Read the model definition and answer for the solid it produces. Units are mm, in the model's axes. A direction names the side the tool comes from. Coordinates: 2 decimals unless noted, no trailing zeros. Write each loop counter-clockwise with the first axis right and the second up, starting at its lowest first coordinate (ties: lowest second). Pieces come first, ordered by that corner, then holes.
(1) Find the intervals of material crossed by probe 1 along X at (y, z) = (-1.5, -0.05); probe 2 along X at (y, z) = (1, -0.35); probe 3 along Z at (x, y) = (-9, -0.5), in increasing order.
(2) Section B-B on y = 1 is taken. Write down the section's boundary in (x, z).
(3) Which of the six approach directions +Z, -Z, +X, -X, +Y, -Y give full straight-line access (tool end or side, diameter ignored) to faces 1 (the flat face through (0, 0, 0)), 2 (the flat face through (0, 0, 1.2))?
(4) Given pin 1 (1.5 mm diameter, centred on x = -18.08, y = 0.47, fed in from +Z), flat-ended and moving along its own axis, determine where the tip first touches the part or whether it passes through.
(5) Section A-A on y = -1.25 is taken. Write down the section's boundary in (x, z), then the cut area to 3 significant figures.
(6) The mould has two halves that part along X. Classify faces 3 (the cylindrical face through (0.295, -4.139, 0.858)), 4 (the cylindrical face through (19.324, 0.525, 0.338)), 5 (the flat face through (-21.5, 0, 0)), 6 (the flat face through (21.5, 0, 0)): +X half, -X half, draft (parallel to the pull), parting line (faces both ways), or undercut.
from build123d import *

# Parameters (mm, degrees)
ESBO_O1_W                = 43
ESBO_O1_H                = 9
RESSALTO_EXTRUS_O1_DEPTH = 1.2
ESBO_O4_W                = 5
ESBO_O4_H                = 9
RESSALTO_EXTRUS_O4_DEPTH = 0.5
FILETE1_R                = 1.2
FILETE2_R                = 1.2
ESBO_O6_R                = 1.25
CORTE_EXTRUS_O2_DEPTH    = 5.5
FILETE3_R                = 0.4
FILETE4_R                = 0.4
ESBO_O7_R                = 0.25
CORTE_EXTRUS_O3_DEPTH    = 23.031568281


with BuildPart() as part:
    # Esboço1 → Ressalto-extrusão1 (new body)
    with BuildSketch(Plane.XY):
        Rectangle(ESBO_O1_W, ESBO_O1_H)
    extrude(amount=RESSALTO_EXTRUS_O1_DEPTH)

    # Esboço4 → Ressalto-extrusão4 (add)
    with BuildSketch(Plane(origin=(0, 0, 0), x_dir=(-1, 0, 0), z_dir=(0, 0, -1))):
        with Locations((19, 0)):
            Rectangle(ESBO_O4_W, ESBO_O4_H)
        with Locations((-19, 0)):
            Rectangle(ESBO_O4_W, ESBO_O4_H)
    extrude(amount=RESSALTO_EXTRUS_O4_DEPTH)

    # Filete1
    filete1_edges = [part.edges().sort_by_distance(p)[0] for p in [
        (0, 4.5, 1.2),
    ]]
    fillet(filete1_edges, radius=FILETE1_R - 0.0001)  # a hair under: the kernel refuses the full size

    # Filete2
    filete2_edges = [part.edges().sort_by_distance(p)[0] for p in [
        (0, -4.5, 1.2),
    ]]
    fillet(filete2_edges, radius=FILETE2_R - 0.0001)  # a hair under: the kernel refuses the full size

    # Esboço6 → Corte-extrusão2 (cut)
    with BuildSketch(Plane(origin=(0, 0, -0.5), x_dir=(-1, 0, 0), z_dir=(0, 0, -1))):
        with Locations((-18.075, 0.470186795)):
            Circle(ESBO_O6_R)
        with Locations((18.075, 0.470186795)):
            Circle(ESBO_O6_R)
    extrude(amount=-CORTE_EXTRUS_O2_DEPTH, mode=Mode.SUBTRACT)

    # Filete3
    filete3_edges = [part.edges().sort_by_distance(p)[0] for p in [
        (-21.5, 0, 1.2),
        (-21.5, 4.5, -0.24995),
        (-21.5, 4.148557427, 0.848557427),
        (-21.5, -4.5, -0.24995),
        (-21.5, -4.148557427, 0.848557427),
    ]]
    fillet(filete3_edges, radius=FILETE3_R)

    # Filete4
    filete4_edges = [part.edges().sort_by_distance(p)[0] for p in [
        (21.5, 4.5, -0.24995),
        (21.5, 4.148557427, 0.848557427),
        (21.5, 0, 1.2),
        (21.5, -4.5, -0.24995),
        (21.5, -4.148557427, 0.848557427),
    ]]
    fillet(filete4_edges, radius=FILETE4_R)

    # Esboço7 → Corte-extrusão3 (cut, through all)
    with BuildSketch(Plane.XY.offset(1.2)):
        with Locations((14.375, -0.529813205)):
            Circle(ESBO_O7_R)
        with Locations((-14.375, -0.529813205)):
            Circle(ESBO_O7_R)
        with Locations((-9.875, -0.529813205)):
            Circle(ESBO_O7_R)
        with Locations((-5.375, -0.529813205)):
            Circle(ESBO_O7_R)
        with Locations((9.875, -0.529813205)):
            Circle(ESBO_O7_R)
        with Locations((5.375, -0.529813205)):
            Circle(ESBO_O7_R)
    extrude(amount=-CORTE_EXTRUS_O3_DEPTH, mode=Mode.SUBTRACT)


solid = part.part
Response:
1. probe 1: x = -21.5 to -16.5, 16.5 to 21.5
1. probe 2: x = -21.5 to -19.21, -16.94 to -16.5, 16.5 to 16.94, 19.21 to 21.5
1. probe 3: z = 0 to 1.2
2. outline: (-21.5, -0.5) - (-19.21, -0.5) - (-19.21, 1.2) - (-21.1, 1.2) arc R0.4 ccw to (-21.5, 0.8) - close; (-16.94, -0.5) - (-16.5, -0.5) - (-16.5, 0) - (16.5, 0) - (16.5, -0.5) - (16.94, -0.5) - (16.94, 1.2) - (-16.94, 1.2) - close; (19.21, -0.5) - (21.5, -0.5) - (21.5, 0.8) arc R0.4 ccw to (21.1, 1.2) - (19.21, 1.2) - close
3. face 1: -Z, +Y, -Y
3. face 2: +Z, +X, -X, +Y, -Y
4. pin 1: passes through
5. outline: (-21.5, -0.5) - (-16.5, -0.5) - (-16.5, 0) - (16.5, 0) - (16.5, -0.5) - (21.5, -0.5) - (21.5, 0.8) arc R0.4 ccw to (21.1, 1.2) - (-21.1, 1.2) arc R0.4 ccw to (-21.5, 0.8) - close
5. area: 56.5 mm2
6. face 3: draft
6. face 4: undercut
6. face 5: -X half
6. face 6: +X half
